Could you check a few things on this model? Use its own coordinates, in mm. A direction names the side the tool comes from. Round coordinates to 2 decimals unless told otherwise and drop trailing zeros. Loops run counter-clockwise (first coordinate to the right, second up) from the corner with the lowest first, then second, coordinate; pieces in that order, holes last. Notation, with made-up numbers: M 73,42.5 L 123,42.5 A11 cw 123,62.5 Z; hole C -35,-21 d10. An arc over 180 degrees is marked long. Answer in a Markdown table with one row per item.
Autodesk Inventor part; units mm, degrees
ref_plane "YZ Plane" through (0, 0, 0) normal (1, 0, 0) x (0, 1, 0)
ref_plane "XZ Plane" through (0, 0, 0) normal (0, 1, 0) x (-1, 0, 0)
ref_plane "XY Plane" through (0, 0, 0) normal (0, 0, 1) x (1, 0, 0)
sketch "スケッチ1" plane through (0, 0, 0) normal (0, 0, 1) x (1, 0, 0)
  circle A0 centre (-17.5, -7.5) radius 1.5
  circle A1 centre (17.5, 7.5) radius 1.5
  circle A2 centre (-17.5, -7.5) radius 4
  circle A3 centre (17.5, 7.5) radius 4
  line L0 (-2.5, -12.5) -> (7.5, -12.5)
  line L1 (7.5, -12.5) -> (7.5, -15.5)
  line L2 (7.5, -15.5) -> (-2.5, -15.5)
  line L3 (-2.5, -15.5) -> (-2.5, -12.5)
  circle A4 centre (-1.4, -12.5) radius 1.1
  line L4 (-2.5, -14) -> (7.5, -14) construction
  line L5 (2.5, -14) -> (2.5, -12.5) construction
  circle A5 centre (-1.4, -15.5) radius 1.1
  circle A6 centre (6.4, -12.5) radius 1.1
  circle A7 centre (6.4, -15.5) radius 1.1
  circle A8 centre (-7.5, -14) radius 1.1
  circle A9 centre (12.5, -14) radius 1.1
  line L6 (-19.0757, -3.8234) -> (15.9243, 11.1766)
  line L7 (21.5, 7.5) -> (21.5, -11.5)
  line L8 (-10, -11.5) -> (21.5, -11.5)
  line L9 (21.5, -11.5) -> (21.5, -16.5)
  line L10 (21.5, -16.5) -> (-10, -16.5)
  line L11 (-10, -16.5) -> (-10, -11.5)
  line L12 (-2.5, -15.5) -> (-2.5, -16.5)
  line L13 (7.5, -15.5) -> (7.5, -16.5)
  line L14 (-17.5, -11.5) -> (-10, -11.5)
  line L15 (21.5, -11.5) -> (21.5, -11.5)
  line L16 (-14.0359, -9.5) -> (19.5, -9.5)
  line L17 (19.5, 4.0359) -> (19.5, -9.5)
  line L18 (-15.1038, -4.2971) -> (13.5281, 7.9737)
  point P0 (0, 0)
  point P1 (-0.3, -12.5)
  point P2 (5.3, -12.5)
  point P3 (7.5, -12.5)
  dimension "d12" = 2.2
  dimension "d0" = 3
  dimension "d1" = 3
  dimension "d2" = 35
  dimension "d5" = 7.5
  dimension "d6" = 15
  dimension "d7" = 17.5
  dimension "d8" = 8
  dimension "d9" = 8
  dimension "d10" = 10
  dimension "d11" = 3
  dimension "d13" = 2.2
  dimension "d14" = 5
  dimension "d15" = 20
  dimension "d19" = 2.5
  dimension "d21" = 1
  dimension "d22" = 2
  dimension "d23" = 2
  dimension "d24" = 2
  dimension "d29" = 5
extrude "押し出し1" add sketch "スケッチ1" along normal blind 1.5 contours A2 | A2 L6 A3 L18 | L16 L17 A3 L7 L8 A6 A4 L14 A2 | A3 | L8 A4 L3 L12 L10 L11 | L9 L10 L13 L1 A6 L8 | L8 A6 L0 A4
fillet "フィレット1" radius 2 8 edges at (-10, -16.5, 0.75) (-10, -11.5, 0.75) (19.5, -9.5, 0.75) (21.5, -16.5, 0.75) (19.5, 4.0359, 0.75) (13.5281, 7.9737, 0.75) (-14.0359, -9.5, 0.75) (-15.1038, -4.2971, 0.75)
equation "\"d8\" = d9"
equation "\"d22\" = d24"
equation "\"d24\" = d23"
properties part number "シン・足首"
1) Will these pins go through, and if not, where does the flat tip stop? P1, Ø3.5, axis at x = 17.5, y = 7.5, coming from the -Z side; P2, Ø0.8, axis at y = -14, z = 1, coming from the -X side; P3, Ø12, axis at x = -14, y = 8, coming from the -Z side; P4, Ø0.8, axis at y = -15, z = 0.5, coming from the +X side.
Computed:
| item | result |
|---|---|
| P1 | stops at z = 0 |
| P2 | stops at x = -10 |
| P3 | passes through |
| P4 | stops at x = 21.5 |
2) I want a section at B-B, the plane x = 3.5. Please give me the cut outline in (y, z).
Computed:
| item | result |
|---|---|
| outline | M -12.5,0 L -9.5,0 L -9.5,1.5 L -12.5,1.5 Z; M 3.68,0 L 5.85,0 L 5.85,1.5 L 3.68,1.5 Z |
3) I need wall thicknesses on line 1 (Y direction, x = 17.5, z = 1.15); line 2 (Y direction, x = 12.5, z = 0.4); line 3 (X direction, y = -5, z = 1.45). Which ranges of each line are inside material? Lowest first, please.
Computed:
| item | result |
|---|---|
| line 1 | y = -16.5 to -9.5, 3.5 to 6, 9 to 11.5 |
| line 2 | y = -16.5 to -15.1, -12.9 to -9.5, 7.07 to 9.71 |
| line 3 | x = -20.62 to -13.98, 19.5 to 21.5 |
4) Which directions (+Z, -Z, +X, -X, +Y, -Y) give clear straight access to the entire face, cutting with the end or side of a thin tool? Please do faces 1 (the face through (7.5, -14, 1)), 2 (the face through (20.9, -15.93, 0.76)), 3 (the face through (19.5, -3, 1)).
Computed:
| item | result |
|---|---|
| face 1 | +Z, -Z, -Y |
| face 2 | +Z, -Z, +X, -Y |
| face 3 | +Z, -Z |
5) I want a section at C-C, the plane x = -7.5. Please give me the cut outline in (y, z), plus the area to 3 significant figures.
Computed:
| item | result |
|---|---|
| outline | M -16.5,0 L -15.1,0 L -15.1,1.5 L -16.5,1.5 Z; M -12.9,0 L -9.5,0 L -9.5,1.5 L -12.9,1.5 Z; M -1.04,0 L 1.14,0 L 1.14,1.5 L -1.04,1.5 Z |
| area | 10.5 mm² |
6) If we mould it in two halves opening along Y, with no side actions, what happens to faces 4 (the face through (-21.4, -8.38, 0.74)), 5 (the face through (18.93, 2.9, 0.76)), 6 (the face through (-10.57, -12.1, 0.76))? For each: released by +Y, released by -Y, zero draft, split by the parting line, or undercut.
Computed:
| item | result |
|---|---|
| face 4 | split by the parting line |
| face 5 | undercut |
| face 6 | released by -Y |
7) I want a section at A-A, the plane y = -12. Please give me the cut outline in (x, z).
Computed:
| item | result |
|---|---|
| outline | M -10.68,0 L -2.38,0 L -2.38,1.5 L -10.68,1.5 Z; M -0.42,0 L 5.42,0 L 5.42,1.5 L -0.42,1.5 Z; M 7.38,0 L 21.5,0 L 21.5,1.5 L 7.38,1.5 Z |
8) I want a section at D-D, the plane y = 1. Please give me the cut outline in (x, z).
Computed:
| item | result |
|---|---|
| outline | M -7.82,0 L -2.74,0 L -2.74,1.5 L -7.82,1.5 Z; M 19.5,0 L 21.5,0 L 21.5,1.5 L 19.5,1.5 Z |
